Work out the finished part from the listing and answer in its coordinate system (mm). A direction names the side the tool comes from. Round coordinates to 2 decimals unless told otherwise and drop trailing zeros. Write each loop counter-clockwise with the first axis right and the second up, starting at its lowest first coordinate (ties: lowest second). Pieces come first, ordered by that corner, then holes. Notation, with made-up numbers: (62.25, 8.5) -> (77.25, 8.5) arc R26 cw to (77.25, 35.5) -> close; hole circle Ø2 at (20.5, 28.5). An arc over 180 degrees is marked (long way). One line per item, written item: value.
```python
from build123d import *

# Parameters (mm, degrees)
BOSS_EXTRUDE2_DEPTH = 9
FILLET1_R           = 0.5
CUT_EXTRUDE1_START  = -5.4
CUT_EXTRUDE1_DEPTH  = 5.4


with BuildPart() as part:
    # Sketch3 → Boss-Extrude2 (new body, symmetric)
    with BuildSketch(Plane(origin=(0, 0, 0), x_dir=(-1, 0, 0), z_dir=(0, -1, 0))):
        with BuildLine():
            Line((-12.669323516, -16.6), (-2.669323516, -16.6))
            Line((-2.669323516, -16.6), (-2.669323516, -16.8))
            ThreePointArc((-2.669323516, -16.8), (-2.962216735, -17.507106781), (-3.669323516, -17.8))
            Line((-3.669323516, -17.8), (-5.669323516, -17.8))
            ThreePointArc((-5.669323516, -17.8), (-8.639171997, -19.030151519), (-9.869323516, -22))
            ThreePointArc((-9.869323516, -22), (-12.669323516, -24.8), (-15.469323516, -22))
            ThreePointArc((-15.469323516, -22), (-16.699475035, -19.030151519), (-19.669323516, -17.8))
            Line((-19.669323516, -17.8), (-21.669323516, -17.8))
            ThreePointArc((-21.669323516, -17.8), (-22.376430297, -17.507106781), (-22.669323516, -16.8))
            Line((-22.669323516, -16.8), (-22.669323516, -16.6))
            Line((-22.669323516, -16.6), (-12.669323516, -16.6))
        make_face()
    extrude(amount=BOSS_EXTRUDE2_DEPTH, both=True)

    # Fillet1
    fillet1_edges = [part.edges().sort_by_distance(p)[0] for p in [
        (22.376430297, -9, 17.507106781),
        (2.669323516, 9, 16.7),
        (2.962216735, 9, 17.507106781),
        (4.669323516, 9, 17.8),
        (8.639171997, 9, 19.030151519),
        (12.669323516, 9, 24.8),
        (16.699475035, 9, 19.030151519),
        (20.669323516, 9, 17.8),
        (20.669323516, -9, 17.8),
        (22.376430297, 9, 17.507106781),
        (22.669323516, 9, 16.7),
        (16.699475035, -9, 19.030151519),
        (12.669323516, -9, 24.8),
        (8.639171997, -9, 19.030151519),
        (4.669323516, -9, 17.8),
        (2.962216735, -9, 17.507106781),
        (2.669323516, -9, 16.7),
        (22.669323516, -9, 16.7),
    ]]
    fillet(fillet1_edges, radius=FILLET1_R)

    # Sketch4 → Cut-Extrude1 (cut)
    with BuildSketch(Plane(origin=(0, 0, 16.6), x_dir=(-1, 0, 0), z_dir=(0, 0, -1)).offset(CUT_EXTRUDE1_START)):
        with BuildLine():
            Line((-14.869323516, 0.8), (-14.869323516, -0.8))
            Line((-14.869323516, -0.8), (-14.769323516, -0.8))
            ThreePointArc((-14.769323516, -0.8), (-14.369323516, -0.6), (-13.969323516, -0.8))
            Line((-13.969323516, -0.8), (-11.369323516, -0.8))
            ThreePointArc((-11.369323516, -0.8), (-10.969323516, -0.6), (-10.569323516, -0.8))
            Line((-10.569323516, -0.8), (-10.469323516, -0.8))
            Line((-10.469323516, -0.8), (-10.469323516, 0.8))
            Line((-10.469323516, 0.8), (-10.569323516, 0.8))
            ThreePointArc((-10.569323516, 0.8), (-10.969323516, 0.6), (-11.369323516, 0.8))
            Line((-11.369323516, 0.8), (-13.969323516, 0.8))
            ThreePointArc((-13.969323516, 0.8), (-14.369323516, 0.6), (-14.769323516, 0.8))
            Line((-14.769323516, 0.8), (-14.869323516, 0.8))
        make_face()
    extrude(amount=CUT_EXTRUDE1_DEPTH, mode=Mode.SUBTRACT)


solid = part.part
```
(1) Consider probe 1 along Y at (x, z) = (14.5, 19.75); probe 2 along Z at (x, y) = (4, -7.75); probe 3 along X at (y, z) = (-1, 22.25). Determine where each line is inside the solid, lowest interval first.
Reported:
probe 1: y = -9 to -0.62, 0.62 to 9
probe 2: z = 16.6 to 17.8
probe 3: x = 9.88 to 15.46
(2) Flat-ended cylindrical pins translate along their axes: pin 1 Ø1.3 at (x, y) = (13.5, 0) entering from -Z; pin 2 Ø1.5 at (y, z) = (-1, 21) entering from +X; pin 3 Ø1.8 at (y, z) = (0.5, 20) entering from -X; pin 4 Ø2 at (x, z) = (17, 24) entering from +Y (3 decimals). Find the tip coordinate at first contact, or state that the pin passes through.
Reported:
pin 1: stops at z = 22
pin 2: stops at x = 15.85
pin 3: stops at x = 8.71
pin 4: passes through
(3) Find section B-B on x = 4.5. Give the vertices of the cut face in (y, z).
Reported:
outline: (-9, 16.6) -> (9, 16.6) -> (9, 17.3) arc R0.5 ccw to (8.5, 17.8) -> (-8.5, 17.8) arc R0.5 ccw to (-9, 17.3) -> close
(4) A tool of negligible diameter and unlimited length cuts with its end or side. For faces 5 (the face through (5, 0, 17.8)), 6 (the face through (13, -2, 16.6)), 7 (the face through (13, 9, 20)), 8 (the face through (13, -0.8, 19)), 9 (the face through (21, 0, 17.8)), from which of +Z, -Z, +X, -X, +Y, -Y can it reach the whole face along a straight path? Write none if from no direction.
Reported:
face 5: +Z, -X, +Y, -Y
face 6: -Z, +X, -X, +Y, -Y
face 7: +Z, -Z, +X, -X, +Y
face 8: -Z
face 9: +Z, +X, +Y, -Y
(5) Find section A-A on y = -2.75. Give the vertices of the cut face in (x, z), plus the area to 3 significant figures.
Reported:
outline: (2.67, 16.6) -> (22.67, 16.6) -> (22.67, 16.8) arc R1 ccw to (21.67, 17.8) -> (19.67, 17.8) arc R4.2 cw to (15.47, 22) arc R2.8 ccw to (9.87, 22) arc R4.2 cw to (5.67, 17.8) -> (3.67, 17.8) arc R1 ccw to (2.67, 16.8) -> close
area: 67.0 mm2
(6) For a pull along X with two mould halves and no side action, classify faces 1 (the face through (2.954, -0.119, 17.499)), 2 (the face through (14.869, 0, 19)), 3 (the face through (13, -9, 20)), 4 (the face through (12.6, -0.1, 24.8)) as pulls with the +X half, pulls with the -X half, needs draft (parallel to the pull), parting line crosses it, or undercut.
Reported:
face 1: pulls with the -X half
face 2: undercut
face 3: needs draft
face 4: parting line crosses it
